The drawing under review shows one solid part. Ordinate dimensions are in mm from its lowest x, y, z. A direction names the side the tool comes from. Round coordinates to 2 decimals unless told otherwise and drop trailing zeros. Write each loop counter-clockwise with the first axis right and the second up, starting at its lowest first coordinate (ties: lowest second). Pieces come first, ordered by that corner, then holes. Notation, with made-up numbers: M 57.25,28.5 L 83.25,28.5 A20 ccw 83.25,38.5 Z; hole C 74.25,-30.5 d3. An arc over 180 degrees is marked long. One line per item, written item: value. Start each with the question number.
1) Wall thickness on probe 1 along X at (y, z) = (9.75, 3.75) (1 decimal); probe 2 along Z at (x, y) = (16, 5.75) (1 decimal); probe 3 along Y at (x, z) = (10.5, 6.25) (1 decimal): over which ranges is each line inside the solid? List them lowest first.
2) Take a section at B-B, the plane y = 4. Write out the cut boundary in (x, z) (1 decimal).
3) Take a section at A-A, the plane z = 7.5. Write out the cut boundary in (x, y) (1 decimal).
4) Tool access review of the marked faces 1, 2 and 3: name each direction out of +Z, -Z, +X, -X, +Y, -Y from which nothing blocks a thin tool from reaching the whole face with its end or side.
5) For P1, Ø4, axis at x = 29.5, z = 9, coming from the -Y side (1 decimal); P2, Ø3, axis at y = 4.5, z = 1.5, coming from the +X side; P3, Ø3, axis at x = 35.5, y = 2.5, coming from the +Z side, all flat-tipped, find the tip position at first contact; note any pin that passes through.
6) Take a section at D-D, the plane z = 2.25. Write out the cut boundary in (x, y) (1 decimal).
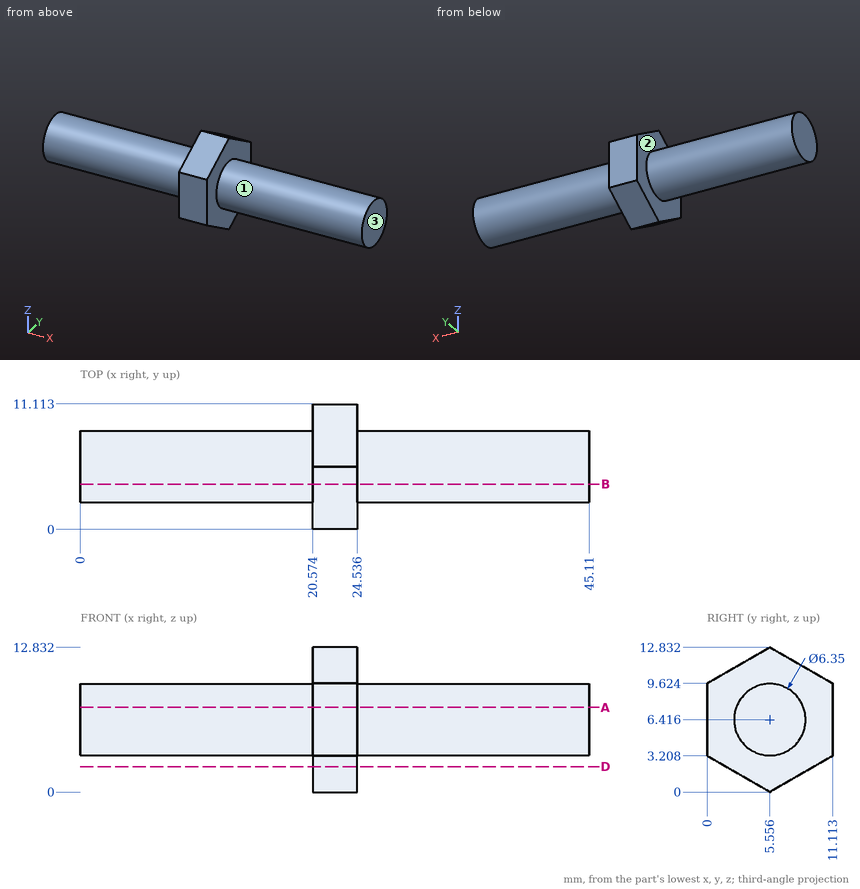
Checked values:
1. probe 1: x = 20.6 to 24.5
1. probe 2: z = 3.2 to 9.6
1. probe 3: y = 2.4 to 8.7
2. outline: M 0,3.6 L 20.6,3.6 L 20.6,0.9 L 24.5,0.9 L 24.5,3.6 L 45.1,3.6 L 45.1,9.2 L 24.5,9.2 L 24.5,11.9 L 20.6,11.9 L 20.6,9.2 L 0,9.2 Z
3. outline: M 0,2.6 L 20.6,2.6 L 20.6,0 L 24.5,0 L 24.5,2.6 L 45.1,2.6 L 45.1,8.5 L 24.5,8.5 L 24.5,11.1 L 20.6,11.1 L 20.6,8.5 L 0,8.5 Z
4. face 1: +X
4. face 2: -X
4. face 3: +Z, -Z, +X, +Y, -Y
5. P1: stops at y = 2.4
5. P2: stops at x = 24.54
5. P3: stops at z = 9.18
6. outline: M 20.6,1.7 L 24.5,1.7 L 24.5,9.5 L 20.6,9.5 Z
